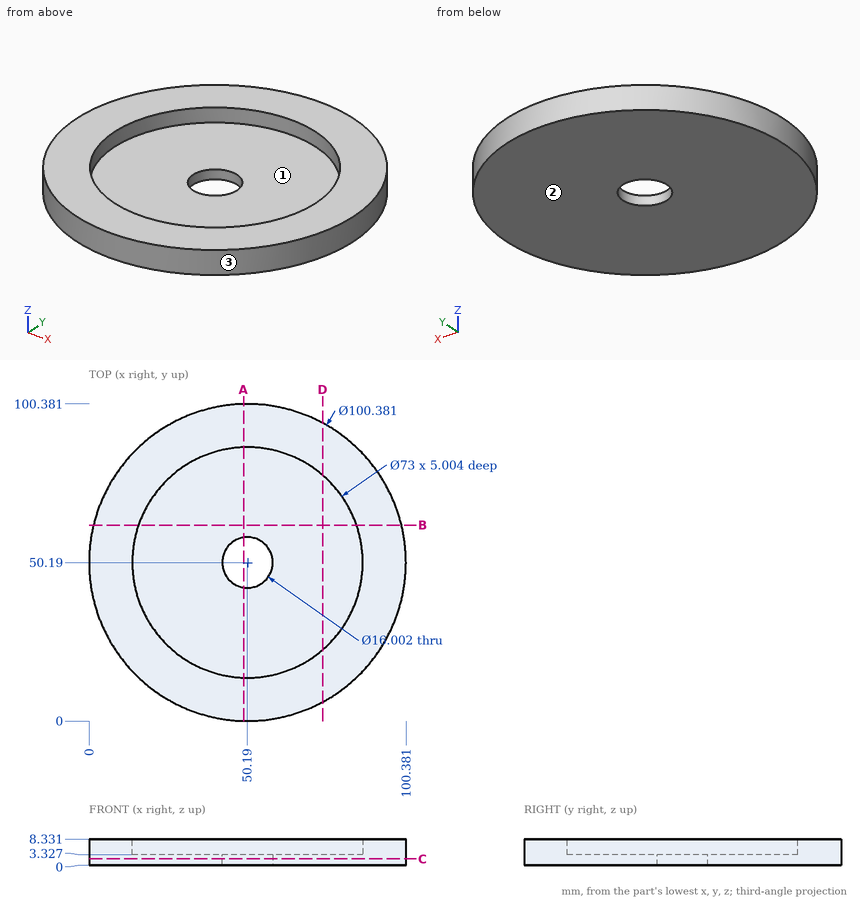
Here's the drawing with two shaded views (mm, measured from the low corner). I have some questions. Give positions to 0.01 mm unless a question says otherwise; leave off trailing zeros. Order: outer loops, then holes, each group sorted by start corner. A loop starts at its lowest first (then second) coordinate and runs counter-clockwise, first axis right, second up.
Q1. Suppose I cut it at A-A, the plane x = 49. Write out the boundary of the cut face in (y, z).
Q2. Suppose I cut it at D-D, the plane x = 74. Write out the boundary of the cut face in (y, z) (1 decimal).
Q3. I'm going to push flat-ended pins straight in: P1, Ø22, axis at x = 60, y = 63, coming from the +Z side; P2, Ø10, axis at x = 65.5, y = 17, coming from the -Z side; P3, Ø4, axis at y = 77, z = 2, coming from the +X side. Where does each tip first touch, or does it pass through?
Q4. Suppose I cut it at C-C, the plane z = 2. Write out the boundary of the cut face in (x, y), and give its area (3 significant figures).
Q5. Suppose I cut it at B-B, the plane y = 62. Write out the boundary of the cut face in (x, z), and give its area (3 significant figures).
Q6. If I drill on line 1 along Z through (x, y) = (65, 68); line 2 along Y through (x, z) = (20.5, 8) (1 decimal); line 3 along X through (y, z) = (65.5, 4.25) (1 decimal), over which ranges is the centre line in solid material (lowest first)?
Q7. We'd pull the mould along X, two halves only. Please class the marked faces 1, 2 and 3: +X half, -X half, draft (parallel to the pull), parting line (faces both ways), or undercut.
Solution:
1. outline: (0.01, 0) - (42.28, 0) - (42.28, 3.33) - (13.71, 3.33) - (13.71, 8.33) - (0.01, 8.33) - close; (58.1, 0) - (100.37, 0) - (100.37, 8.33) - (86.67, 8.33) - (86.67, 3.33) - (58.1, 3.33) - close
2. outline: (6, 0) - (94.4, 0) - (94.4, 8.3) - (77.9, 8.3) - (77.9, 3.3) - (22.5, 3.3) - (22.5, 8.3) - (6, 8.3) - close
3. P1: stops at z = 3.33
3. P2: stops at z = 0
3. P3: stops at x = 93.82
4. outline: circle Ø100.38 at (50.19, 50.19); hole circle Ø16 at (50.19, 50.19)
4. area: 7,710 mm2
5. outline: (1.41, 0) - (98.97, 0) - (98.97, 8.33) - (84.73, 8.33) - (84.73, 3.33) - (15.65, 3.33) - (15.65, 8.33) - (1.41, 8.33) - close
5. area: 467 mm2
6. line 1: z = 0 to 3.33
6. line 2: y = 9.7 to 29, 71.4 to 90.7
6. line 3: x = 2.4 to 17.1, 83.3 to 98
7. face 1: undercut
7. face 2: draft
7. face 3: parting line
